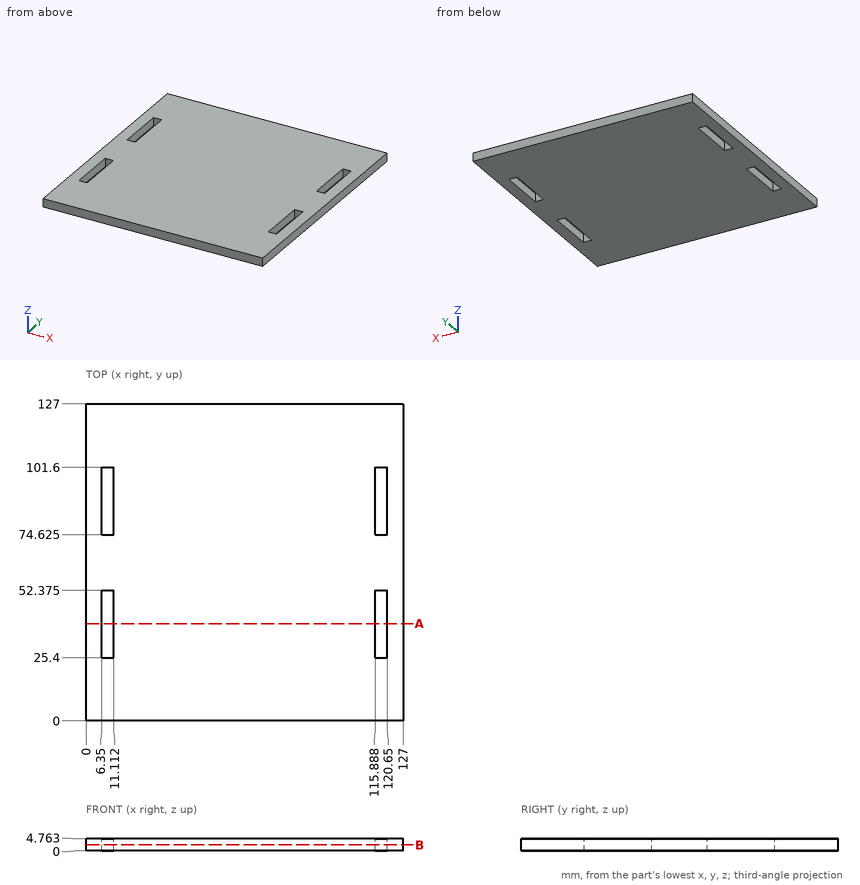
Check sheet for the drawn part. Datum: minimum x, y, z corner. Units: mm. Give positions to 0.01 mm unless a question says otherwise; leave off trailing zeros. Loops run counter-clockwise (first coordinate to the right, second up) from the corner with the lowest first, then second, coordinate; pieces in that order, holes last. Notation, with made-up numbers: M 80.5,57.5 L 94.5,57.5 A10 ccw 94.5,66.5 Z; hole C 48.25,11 d1. An arc over 180 degrees is marked long. Answer as CSV lines item,"result".
Item 1: Sectioned sample at A-A, the plane y = 39. Enter the section's corners in (x, z).
Reply:
outline,"M 0,0 L 6.35,0 L 6.35,4.76 L 0,4.76 Z; M 11.11,0 L 115.89,0 L 115.89,4.76 L 11.11,4.76 Z; M 120.65,0 L 127,0 L 127,4.76 L 120.65,4.76 Z"
Item 2: Scan line: L1, parallel to X at y = 34.5, z = 2.5. Record every from-to range of solid material in increasing order.
Reply:
L1,"0 to 6.35, 11.11 to 115.89, 120.65 to 127"
Item 3: Sectioned sample at B-B, the plane z = 2.4. State how many separate pieces and enclosed holes the cut face has, then the cut area to 3 significant figures.
Reply:
separate pieces,"1"
enclosed holes,"4"
area,"15,600 mm^2"
Item 4: Depth check by flat-ended pin: pin 1 Ø1.4 at (x, z) = (119, 3.5) entering from -Y. Enter the tip coordinate at first touch or a pass-through.
Reply:
pin 1,"y = 0"
